Geometry check sheet. Reference: the model listing, model coordinates, mm. Give positions to 0.01 mm unless a question says otherwise; leave off trailing zeros. Loops run counter-clockwise (first coordinate to the right, second up) from the corner with the lowest first, then second, coordinate; pieces in that order, holes last. Notation, with made-up numbers: (-8.5, -35.75) -> (24.5, -35.75) arc R17 cw to (24.5, -27.75) -> close; hole circle Ø11 at (4, -10). An arc over 180 degrees is marked (long way). Write item = value, one per line.
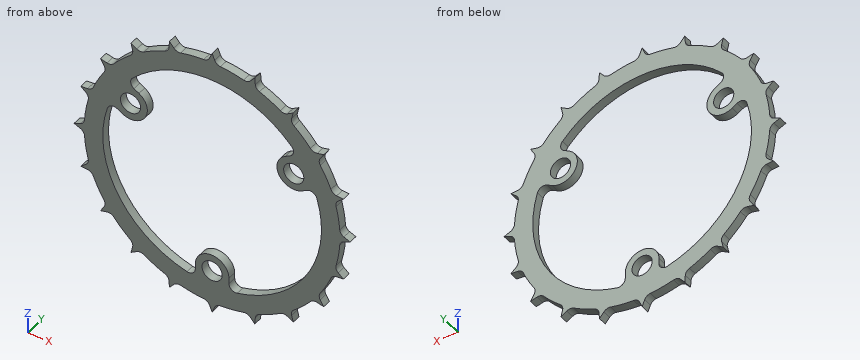
```python
from build123d import *

# Parameters (mm, degrees)
SKETCH1_R                = 24.13
BOSS_EXTRUDE1_DEPTH      = 0.8001
BOSS_EXTRUDE2_DEPTH      = 1.6002
FILLET1_R                = 1.27
CIRPATTERN1_COUNT        = 20
FILLET1_OF_CIRPATTERN1_R = 1.27
SKETCH3_R                = 20.6375
CUT_EXTRUDE1_DEPTH       = 2.6002
SKETCH4_R                = 1.905
BOSS_EXTRUDE3_DEPTH      = 1.6002
FILLET2_R                = 1.27
CIRPATTERN2_COUNT        = 3
FILLET2_OF_CIRPATTERN2_R = 1.27


with BuildPart() as part:
    # Sketch1 → Boss-Extrude1 (new body, symmetric)
    with BuildSketch(Plane(origin=(0, 0, 0), x_dir=(1, 0, 0), z_dir=(0, 1, 0))):
        Circle(SKETCH1_R)
    extrude(amount=BOSS_EXTRUDE1_DEPTH, both=True)

    # Sketch2 → Boss-Extrude2 (add, through all)
    with BuildSketch(Plane(origin=(0, 0.8001, 0), x_dir=(1, 0, 0), z_dir=(0, 1, 0))):
        Polygon((-0.794496075, 24.116916801), (0, 26.035), (0.794496075, 24.116916801), align=None)
    boss_extrude2 = extrude(amount=-BOSS_EXTRUDE2_DEPTH)

    # Fillet1
    fillet1_edges = [part.edges().sort_by_distance(p)[0] for p in [
        (0.794496075, 0, -24.116916801),
        (-0.794496075, 0, -24.116916801),
    ]]
    fillet(fillet1_edges, radius=FILLET1_R)

    # CirPattern1: Boss-Extrude2 ×20 about axis
    cirpattern1_axis = Axis((0, 0, 0), (0, 1, 0))
    for i in range(1, CIRPATTERN1_COUNT):
        add(boss_extrude2.rotate(cirpattern1_axis, i * 360 / CIRPATTERN1_COUNT))

    # Fillet1 of CirPattern1
    fillet1_of_cirpattern1_edges = [part.edges().sort_by_distance(p)[0] for p in [
        (-6.696926474, 0, -23.182063666),
        (-8.208147813, 0, -22.691038087),
        (-13.5328072, 0, -19.97798862),
        (-14.818328853, 0, -19.044002468),
        (-19.044002468, 0, -14.818328853),
        (-19.97798862, 0, -13.5328072),
        (-22.691038087, 0, -8.208147813),
        (-23.182063666, 0, -6.696926474),
        (-24.116916801, 0, -0.794496075),
        (-24.116916801, 0, 0.794496075),
        (-23.182063666, 0, 6.696926474),
        (-22.691038087, 0, 8.208147813),
        (-19.97798862, 0, 13.5328072),
        (-19.044002468, 0, 14.818328853),
        (-14.818328853, 0, 19.044002468),
        (-13.5328072, 0, 19.97798862),
        (-8.208147813, 0, 22.691038087),
        (-6.696926474, 0, 23.182063666),
        (-0.794496075, 0, 24.116916801),
        (0.794496075, 0, 24.116916801),
        (6.696926474, 0, 23.182063666),
        (8.208147813, 0, 22.691038087),
        (13.5328072, 0, 19.97798862),
        (14.818328853, 0, 19.044002468),
        (19.044002468, 0, 14.818328853),
        (19.97798862, 0, 13.5328072),
        (22.691038087, 0, 8.208147813),
        (23.182063666, 0, 6.696926474),
        (24.116916801, 0, 0.794496075),
        (24.116916801, 0, -0.794496075),
        (23.182063666, 0, -6.696926474),
        (22.691038087, 0, -8.208147813),
        (19.97798862, 0, -13.5328072),
        (19.044002468, 0, -14.818328853),
        (14.818328853, 0, -19.044002468),
        (13.5328072, 0, -19.97798862),
        (8.208147813, 0, -22.691038087),
        (6.696926474, 0, -23.182063666),
    ]]
    fillet(fillet1_of_cirpattern1_edges, radius=FILLET1_OF_CIRPATTERN1_R)

    # Sketch3 → Cut-Extrude1 (cut, through all)
    with BuildSketch(Plane(origin=(0, 0.8001, 0), x_dir=(1, 0, 0), z_dir=(0, 1, 0))):
        Circle(SKETCH3_R)
    extrude(amount=-CUT_EXTRUDE1_DEPTH, mode=Mode.SUBTRACT)

    # Sketch4 → Boss-Extrude3 (add, through all)
    with BuildSketch(Plane(origin=(0, 0.8001, 0), x_dir=(1, 0, 0), z_dir=(0, 1, 0))):
        with BuildLine():
            Line((-3.175, 17.78), (-3.175, 20.391806719))
            ThreePointArc((-3.175, 20.391806719), (0, 20.6375), (3.175, 20.391806719))
            Line((3.175, 20.391806719), (3.175, 17.78))
            ThreePointArc((3.175, 17.78), (0, 14.605), (-3.175, 17.78))
        make_face()
        with Locations((0, 17.78)):
            Circle(SKETCH4_R, mode=Mode.SUBTRACT)
    boss_extrude3 = extrude(amount=-BOSS_EXTRUDE3_DEPTH)

    # Fillet2
    fillet2_edges = [part.edges().sort_by_distance(p)[0] for p in [
        (-3.175, 0, -20.391806719),
        (3.175, 0, -20.391806719),
    ]]
    fillet(fillet2_edges, radius=FILLET2_R)

    # CirPattern2: Boss-Extrude3 ×3 about axis
    cirpattern2_axis = Axis((0, 0, 0), (0, 1, 0))
    for i in range(1, CIRPATTERN2_COUNT):
        add(boss_extrude3.rotate(cirpattern2_axis, i * 360 / CIRPATTERN2_COUNT))

    # Fillet2 of CirPattern2
    fillet2_of_cirpattern2_edges = [part.edges().sort_by_distance(p)[0] for p in [
        (-16.072322647, 0, 12.945534016),
        (-19.247322647, 0, 7.446272702),
        (19.247322647, 0, 7.446272702),
        (16.072322647, 0, 12.945534016),
    ]]
    fillet(fillet2_of_cirpattern2_edges, radius=FILLET2_OF_CIRPATTERN2_R)


solid = part.part
```
Item 1: Gauge pin test, flat ends, axial feed: pin 1 (3 mm diameter, centred on x = 0, z = -17.78, fed in from +Y); pin 2 (0.5 mm diameter, centred on y = 0, z = -18.5, fed in from +X). Record the tip position at first contact, or that the pin passes through.
Answer:
pin_1 = through
pin_2 = 15.79
Item 2: Thickness scan on L1, parallel to Z at x = 14, y = 0.35; L2, parallel to X at y = 0.2, z = -18 (3 decimals); L3, parallel to X at y = 0.4, z = 10. Record the ranges inside material, lowest first. Write a range as [from, to].
Answer:
L1 = [-20.29, -15.16], [6.04, 7.6], [10.18, 11.75], [15.16, 20.29]
L2 = [-16.07, -10.095], [-3.175, -1.892], [1.892, 3.175], [10.095, 16.07]
L3 = [-21.96, -16.95], [-13.85, -12.42], [12.42, 13.85], [16.95, 21.96]
Item 3: Section check B-B, the plane y = 0.55. Give the number of separate pieces and of enclosed holes in the cut face, plus the area to 3 significant figures.
Answer:
separate_pieces = 1
enclosed_holes = 4
area = 595 mm^2
Item 4: Section check A-A, the plane x = -10. Record the cut outline in (y, z), plus the area to 3 significant figures.
Answer:
outline = (-0.8, -21.96) -> (0.8, -21.96) -> (0.8, -18.05) -> (-0.8, -18.05) -> close; (-0.8, 18.05) -> (0.8, 18.05) -> (0.8, 21.96) -> (-0.8, 21.96) -> close
area = 12.5 mm^2
